```python
from build123d import *

# Parameters (mm, degrees)
F3_DEPTH      = 38.1
F3_DEPTH_BACK = 38.1


with BuildPart() as f2:
    # F1 (on Front) → F2 (revolve)
    with BuildSketch(Plane.XZ):
        Polygon((-25.4309553104, 8.369750945), (-25.4309553104, 6.464750945), (25.3690446896, 6.464750945), (25.3690446896, 8.369750945), (12.6690446896, 11.544750945), (-12.7309553104, 11.544750945), align=None)
    revolve(axis=Axis((-0.4450748034, 0, 0.114750945), (1, 0, 0)))

    # F0 (on Right) → F3 (cut, two sides)
    with BuildSketch(Plane.YZ) as f3_sk:
        Polygon((7.2894281006, 0.7921939781), (2.9586539406, 6.7089269033), (-4.3307741601, 5.9167329252), (-7.2894281006, -0.7921939781), (-2.9586539406, -6.7089269033), (4.3307741601, -5.9167329252), align=None)
    extrude(amount=-F3_DEPTH, mode=Mode.SUBTRACT)
    extrude(f3_sk.sketch, amount=F3_DEPTH_BACK, mode=Mode.SUBTRACT)


solid = f2.part
```
Input: part model. Units: mm. Frame: model coordinates. A direction names the side the tool comes from. Give positions to 0.01 mm unless a question says otherwise; leave off trailing zeros. Write each loop counter-clockwise with the first axis right and the second up, starting at its lowest first coordinate (ties: lowest second). Pieces come first, ordered by that corner, then holes. Notation, with made-up numbers: (79, -10) - (137, -10) arc R23 ccw to (137, 22) - close; hole circle Ø3 at (6, -23.5). An arc over 180 degrees is marked (long way). Write item = value, one per line. Start each with the question number.
1) Pin query (flat end, axial travel): pin 1 (1.5 mm diameter, centred on x = 9.5, y = -7.5, fed in from +Z); pin 2 (1.5 mm diameter, centred on x = -16.5, y = -4.5, fed in from -Z); pin 3 (5 mm diameter, centred on x = 10.5, z = -3, fed in from -Y); pin 4 (1.5 mm diameter, centred on y = -3.5, z = -4, fed in from -X). Return the tip coordinate at first contact, or that it passes through.
2) Cut plane A-A (x = -9.5). Return loops of the section in (y, z), and give its area (3 significant figures).
3) Cut plane B-B (y = 0). Return loops of the section in (x, z).
4) Cut plane C-C (x = -20.5). Return loops of the section in (y, z), and give its area (3 significant figures).
5) Material intervals for L1, parallel to Z at x = 2, y = -6.5; L2, parallel to Y at x = -7.5, z = -4.75; L3, parallel to Y at x = -20, z = -3.5, sorted ascending. Write a range as [from, to].
6) Draft query along Z for faces 1 (the face through (-21.992, -9.037, -1.072)), 2 (the face through (0.325, -4.887, 4.656)), 3 (the face through (-25.431, 4.9, 4.4)). Return one class per face: pulls with the +Z half, pulls with the -Z half, needs draft (parallel to the pull), parting line crosses it, or undercut.
7) Reachability of faces 4 (the face through (21.752, 8.941, -1.871)), 5 (the face through (0.32, 5.79, -2.61)) from +Z, -Z, +X, -X, +Y, -Y: full face, straight path, thin tool, end or side. Return the list, or none.
Answers follow:
q1.pin_1 = 9.34
q1.pin_2 = -9.74
q1.pin_3 = -11.41
q1.pin_4 = through
q2.outline = circle Ø22.86 at (0, 0.11); hole (-7.29, -0.79) - (-2.96, -6.71) - (4.33, -5.92) - (7.29, 0.79) - (5.62, 3.08) arc R6.35 ccw to (4.52, 4.57) - (2.96, 6.71) - (0.52, 6.44) arc R6.35 ccw to (-1.86, 6.18) - (-4.33, 5.92) - (-5.46, 3.36) arc R6.35 ccw to (-6.08, 1.96) - close
q2.area = 270 mm^2
q3.outline = (-25.43, -8.14) - (-12.73, -11.32) - (12.67, -11.32) - (25.37, -8.14) - (25.37, -6.39) - (-25.43, -6.39) - close; (-25.43, 6.46) - (25.37, 6.46) - (25.37, 8.37) - (12.67, 11.54) - (-12.73, 11.54) - (-25.43, 8.37) - close
q4.outline = circle Ø18.98 at (0, 0.11); hole (-7.29, -0.79) - (-2.96, -6.71) - (4.33, -5.92) - (7.29, 0.79) - (5.62, 3.08) arc R6.35 ccw to (4.52, 4.57) - (2.96, 6.71) - (0.52, 6.44) arc R6.35 ccw to (-1.86, 6.18) - (-4.33, 5.92) - (-5.46, 3.36) arc R6.35 ccw to (-6.08, 1.96) - close
q4.area = 143 mm^2
q5.L1 = [-9.29, -1.87], [1, 9.52]
q5.L2 = [-10.34, -4.39], [4.85, 10.34]
q5.L3 = [-8.91, -5.31], [5.4, 8.91]
q6.face_1 = parting line crosses it
q6.face_2 = undercut
q6.face_3 = needs draft
q7.face_4 = +X
q7.face_5 = +X, -X
